For this review, take the finished solid that the model builds, in its own axes (mm). A direction names the side the tool comes from. Coordinates: 2 decimals unless noted, no trailing zeros. Loops run counter-clockwise (first coordinate to the right, second up) from the corner with the lowest first, then second, coordinate; pieces in that order, holes last.
1. Mouldability with a two-part tool opening along Y and no side actions: class faces 1 (the face through (-36, 36, 3)), 2 (the face through (-46, 90, 1)), 3 (the face through (-37, 45, 1)) as pulls with the +Y half, pulls with the -Y half, needs draft (parallel to the pull), parting line crosses it, or undercut.
2. Take a section at C-C, the plane z = 2.25. State the section outline as (x, y) points, then the cut area to 3 significant figures.
3. Take a section at D-D, the plane x = -18.5. State the section outline as (y, z) points.
4. Take a section at A-A, the plane y = 23. State the section outline as (x, z) points.
5. Take a section at B-B, the plane x = -41.5. State the section outline as (y, z) points.
6. To check wall thickness, follow probe 1 along X at (y, z) = (48.5, 2.2); probe 2 along X at (y, z) = (67, 2.1); probe 3 along Y at (x, z) = (-54, 2.3). State the ranges of each line that lie inside material, in increasing order.
7. Machinability: for faces 4 (the face through (-90, 44, 1)), 5 (the face through (-45, 68, 1)), which of the approach directions +Z, -Z, +X, -X, +Y, -Y give a long, thin tool a straight path to every point of the face, cutting with its end or side? Answer none if there is none.
```python
from build123d import *

# Parameters (mm, degrees)
SKETCH_W     = 90
SKETCH_H     = 90
PAD_DEPTH    = 3
POCKET_DEPTH = 3


with BuildPart() as part:
    # Sketch → Pad (new body)
    with BuildSketch(Plane.XY):
        with Locations((-45, 45)):
            Rectangle(SKETCH_W, SKETCH_H)
    extrude(amount=PAD_DEPTH)

    # Sketch001 (on Face5 of Pad) → Pocket (cut)
    with BuildSketch(Plane(origin=(0, 0, 0), x_dir=(1, 0, 0), z_dir=(0, 0, -1))):
        Polygon((-60, -15), (-60, -30), (-75, -30), (-75, -45), (-60, -45), (-60, -75), (-45, -75), (-45, -60), (-30, -60), (-30, -45), (-45, -45), (-45, -30), (-15, -30), (-15, -15), align=None)
    extrude(amount=-POCKET_DEPTH, mode=Mode.SUBTRACT)


solid = part.part
```
Results list:
1. face 1: needs draft
1. face 2: pulls with the +Y half
1. face 3: undercut
2. outline: (-90, 0) - (0, 0) - (0, 90) - (-90, 90) - close; hole (-75, 30) - (-60, 30) - (-60, 15) - (-15, 15) - (-15, 30) - (-45, 30) - (-45, 45) - (-30, 45) - (-30, 60) - (-45, 60) - (-45, 75) - (-60, 75) - (-60, 45) - (-75, 45) - close
2. area: 6,300 mm2
3. outline: (0, 0) - (15, 0) - (15, 3) - (0, 3) - close; (30, 0) - (90, 0) - (90, 3) - (30, 3) - close
4. outline: (-90, 0) - (-60, 0) - (-60, 3) - (-90, 3) - close; (-15, 0) - (0, 0) - (0, 3) - (-15, 3) - close
5. outline: (0, 0) - (15, 0) - (15, 3) - (0, 3) - close; (30, 0) - (45, 0) - (45, 3) - (30, 3) - close; (60, 0) - (90, 0) - (90, 3) - (60, 3) - close
6. probe 1: x = -90 to -60, -30 to 0
6. probe 2: x = -90 to -60, -45 to 0
6. probe 3: y = 0 to 15, 75 to 90
7. face 4: +Z, -Z, -X, +Y, -Y
7. face 5: +Z, -Z
